Read the model definition and answer for the solid it produces. Units are mm, in the model's axes. Face numbers are marked on the shaded views. A direction names the side the tool comes from. Coordinates: 2 decimals unless noted, no trailing zeros. Order: outer loops, then holes, each group sorted by start corner. A loop starts at its lowest first (then second) coordinate and runs counter-clockwise, first axis right, second up. Notation, with made-up numbers: (88, 26) -> (93, 26) arc R17 ccw to (93, 47) -> close; hole circle Ø3 at (19, 3). An arc over 180 degrees is marked (long way). Answer as a JSON object with one key per item and string values. Group by question number.
1) Section B-B on x = 22.5 is taken. Determine the outline of the cut face in (y, z).
2) A tool of negligible diameter and unlimited length cuts with its end or side. For the marked faces 1 and 2, from which of +Z, -Z, +X, -X, +Y, -Y can it reach the whole face along a straight path? Write none if from no direction.
3) Consider L1, parallel to X at y = 2, z = -66; L2, parallel to X at y = 1.4, z = -45.5; L3, parallel to X at y = 1.35, z = -13.5. Determine where each line is inside the solid, lowest interval first.
4) Section A-A on z = -48 is taken. Determine the outline of the cut face in (x, y).
5) Section D-D on z = -73 is taken. Determine the outline of the cut face in (x, y), and give its area (3 significant figures).
6) Section C-C on y = 0.65 is taken. Determine the outline of the cut face in (x, z).
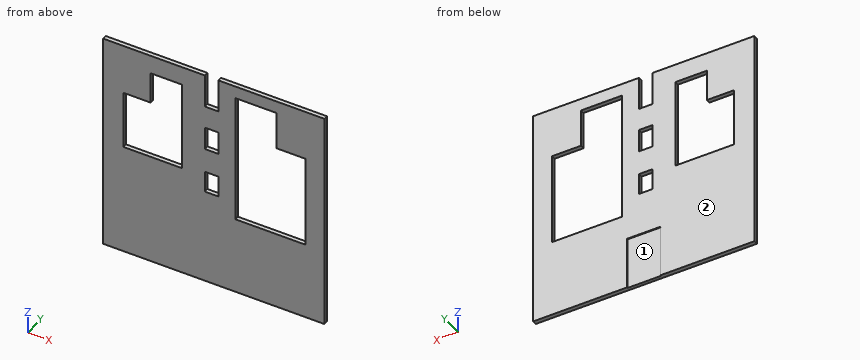
from build123d import *

# Parameters (mm, degrees)
SKETCH1_W           = 120
SKETCH1_H           = 120
BOSS_EXTRUDE1_DEPTH = 2.3
CUT_EXTRUDE1_REACH  = 171.721
SKETCH2_W           = 7.422122634
SKETCH2_H           = 18.177961541
SKETCH2_H_2         = 12.498339484
SKETCH2_H_3         = 11.613798671
SKETCH2_3_W         = 18.1
SKETCH2_3_H         = 28.4
CUT_EXTRUDE2_DEPTH  = 0.5


with BuildPart() as part:
    # Sketch1 → Boss-Extrude1 (new body)
    with BuildSketch(Plane(origin=(0, 0, 0), x_dir=(1, 0, 0), z_dir=(0, 1, 0))):
        with Locations((60, 60)):
            Rectangle(SKETCH1_W, SKETCH1_H)
    extrude(amount=BOSS_EXTRUDE1_DEPTH)

    # Sketch2 → Cut-Extrude1 (cut, up to next)
    with BuildSketch(Plane(origin=(0, 2.3, 0), x_dir=(1, 0, 0), z_dir=(0, 1, 0)), mode=Mode.PRIVATE) as cut_extrude1_sk1:
        Polygon((42.897324416, 59.05835662), (10.950631269, 59.05835662), (10.950631269, 27.396794206), (25.719897068, 27.396794206), (25.719897068, 10.210582129), (42.897324416, 10.210582129), align=None)
    cut_extrude1_tool1 = extrude(cut_extrude1_sk1.sketch, amount=-CUT_EXTRUDE1_REACH, mode=Mode.PRIVATE) & part.part
    # Sketch2 → Cut-Extrude1 (cut, up to next)
    with BuildSketch(Plane(origin=(0, 2.3, 0), x_dir=(1, 0, 0), z_dir=(0, 1, 0)), mode=Mode.PRIVATE) as cut_extrude1_sk2:
        Polygon((109.790535643, 77.620899486), (71.695725531, 77.620899486), (71.695725531, 6.770353139), (94.080420097, 6.770353139), (94.080420097, 27.396794206), (109.790535643, 27.396794206), align=None)
    cut_extrude1_tool2 = extrude(cut_extrude1_sk2.sketch, amount=-CUT_EXTRUDE1_REACH, mode=Mode.PRIVATE) & part.part
    # Sketch2 → Cut-Extrude1 (cut, up to next)
    with BuildSketch(Plane(origin=(0, 2.3, 0), x_dir=(1, 0, 0), z_dir=(0, 1, 0)), mode=Mode.PRIVATE) as cut_extrude1_sk3:
        with Locations((58.912993536, 9.088980771)):
            Rectangle(SKETCH2_W, SKETCH2_H)
    cut_extrude1_tool3 = extrude(cut_extrude1_sk3.sketch, amount=-CUT_EXTRUDE1_REACH, mode=Mode.PRIVATE) & part.part
    # Sketch2 → Cut-Extrude1 (cut, up to next)
    with BuildSketch(Plane(origin=(0, 2.3, 0), x_dir=(1, 0, 0), z_dir=(0, 1, 0)), mode=Mode.PRIVATE) as cut_extrude1_sk4:
        with Locations((58.912993536, 36.747395539)):
            Rectangle(SKETCH2_W, SKETCH2_H_2)
    cut_extrude1_tool4 = extrude(cut_extrude1_sk4.sketch, amount=-CUT_EXTRUDE1_REACH, mode=Mode.PRIVATE) & part.part
    # Sketch2 → Cut-Extrude1 (cut, up to next)
    with BuildSketch(Plane(origin=(0, 2.3, 0), x_dir=(1, 0, 0), z_dir=(0, 1, 0)), mode=Mode.PRIVATE) as cut_extrude1_sk5:
        with Locations((58.912993536, 62.090548619)):
            Rectangle(SKETCH2_W, SKETCH2_H_3)
    cut_extrude1_tool5 = extrude(cut_extrude1_sk5.sketch, amount=-CUT_EXTRUDE1_REACH, mode=Mode.PRIVATE) & part.part
    add(cut_extrude1_tool1.solids().sort_by_distance((28.592347, 2.3, -37.709621))[0], mode=Mode.SUBTRACT)
    add(cut_extrude1_tool2.solids().sort_by_distance((89.216049, 2.3, -45.62191))[0], mode=Mode.SUBTRACT)
    add(cut_extrude1_tool3.solids().sort_by_distance((58.912994, 2.3, -9.088981))[0], mode=Mode.SUBTRACT)
    add(cut_extrude1_tool4.solids().sort_by_distance((58.912994, 2.3, -36.747396))[0], mode=Mode.SUBTRACT)
    add(cut_extrude1_tool5.solids().sort_by_distance((58.912994, 2.3, -62.090549))[0], mode=Mode.SUBTRACT)

    # Sketch2<3> → Cut-Extrude2 (cut)
    with BuildSketch(Plane(origin=(0, 2.3, 0), x_dir=(1, 0, 0), z_dir=(0, 1, 0))):
        with Locations((60, 105.8)):
            Rectangle(SKETCH2_3_W, SKETCH2_3_H)
    extrude(amount=-CUT_EXTRUDE2_DEPTH, mode=Mode.SUBTRACT)


solid = part.part
Worked answers:
{
 "1": {"outline": "(0, -120) -> (2.3, -120) -> (2.3, -59.06) -> (0, -59.06) -> close; (0, -27.4) -> (2.3, -27.4) -> (2.3, 0) -> (0, 0) -> close"},
 "2": {"face 1": "-Z, +Y", "face 2": "+Z, -Z, +X, -X, +Y"},
 "3": {"L1": "x = 0 to 55.2, 62.62 to 71.7, 109.79 to 120", "L2": "x = 0 to 10.95, 42.9 to 71.7, 109.79 to 120", "L3": "x = 0 to 25.72, 42.9 to 55.2, 62.62 to 71.7, 94.08 to 120"},
 "4": {"outline": "(0, 0) -> (10.95, 0) -> (10.95, 2.3) -> (0, 2.3) -> close; (42.9, 0) -> (71.7, 0) -> (71.7, 2.3) -> (42.9, 2.3) -> close; (109.79, 0) -> (120, 0) -> (120, 2.3) -> (109.79, 2.3) -> close"},
 "5": {"outline": "(0, 0) -> (71.7, 0) -> (71.7, 2.3) -> (0, 2.3) -> close; (109.79, 0) -> (120, 0) -> (120, 2.3) -> (109.79, 2.3) -> close", "area": "188 mm²"},
 "6": {"outline": "(0, -120) -> (120, -120) -> (120, 0) -> (62.62, 0) -> (62.62, -18.18) -> (55.2, -18.18) -> (55.2, 0) -> (0, 0) -> close; hole (10.95, -59.06) -> (42.9, -59.06) -> (42.9, -10.21) -> (25.72, -10.21) -> (25.72, -27.4) -> (10.95, -27.4) -> close; hole (55.2, -67.9) -> (62.62, -67.9) -> (62.62, -56.28) -> (55.2, -56.28) -> close; hole (55.2, -43) -> (62.62, -43) -> (62.62, -30.5) -> (55.2, -30.5) -> close; hole (71.7, -77.62) -> (109.79, -77.62) -> (109.79, -27.4) -> (94.08, -27.4) -> (94.08, -6.77) -> (71.7, -6.77) -> close"}
}
